from build123d import *

# Parameters (mm, degrees)
SKETCH1_R           = 40
BOSS_EXTRUDE1_DEPTH = 10
CUT_EXTRUDE1_DEPTH  = 4
SKETCH3_W           = 4
SKETCH3_H           = 15
CUT_EXTRUDE2_DEPTH  = 10


with BuildPart() as part:
    # Sketch1 → Boss-Extrude1 (new body)
    with BuildSketch(Plane(origin=(0, 0, 0), x_dir=(1, 0, 0), z_dir=(0, 1, 0))):
        with Locations(Location((0, 0, 0), (0, 0, 270))):
            Circle(SKETCH1_R)
    extrude(amount=BOSS_EXTRUDE1_DEPTH)

    # Sketch2 → Cut-Extrude1 (cut)
    with BuildSketch(Plane(origin=(0, 10, 0), x_dir=(1, 0, 0), z_dir=(0, 1, 0))):
        with BuildLine():
            Line((-2, 16.764144262), (-3.580103784, 0.764144262))
            ThreePointArc((-3.580103784, 0.764144262), (0, -3.596740326), (3.580103784, 0.764144262))
            Line((3.580103784, 0.764144262), (2, 16.764144262))
            ThreePointArc((2, 16.764144262), (0, 18.764144262), (-2, 16.764144262))
        make_face()
    extrude(amount=-CUT_EXTRUDE1_DEPTH, mode=Mode.SUBTRACT)

    # Sketch3 → Cut-Extrude2 (cut)
    with BuildSketch(Plane.XZ):
        with Locations((13, 0)):
            Rectangle(SKETCH3_W, SKETCH3_H)
        with Locations((-13, 0)):
            Rectangle(SKETCH3_W, SKETCH3_H)
    extrude(amount=-CUT_EXTRUDE2_DEPTH, mode=Mode.SUBTRACT)


solid = part.part
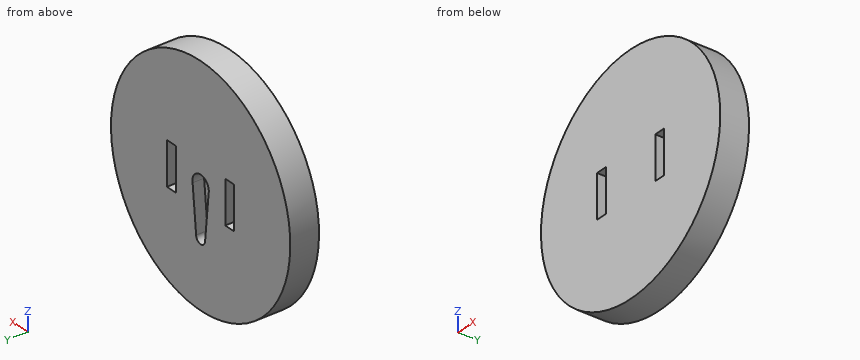
Read the model definition and answer for the solid it produces. Units are mm, in the model's axes. Coordinates: 2 decimals unless noted, no trailing zeros. Write each loop counter-clockwise with the first axis right and the second up, starting at its lowest first coordinate (ties: lowest second). Pieces come first, ordered by that corner, then holes. Notation, with made-up numbers: (29, -36) - (67, -36) arc R21 ccw to (67, -7) - close; hole circle Ø6 at (-3, 4). An arc over 180 degrees is marked (long way). One line per question, with ' | ' between items.
Q1. Find section D-D, the plane z = -5.5. Write down the section's boundary in (x, y), plus the area to 3 significant figures.
Result set:
outline: (-39.62, 0) - (-15, 0) - (-15, 10) - (-39.62, 10) - close; (-11, 0) - (11, 0) - (11, 10) - (3.11, 10) - (3.11, 6) - (-3.11, 6) - (-3.11, 10) - (-11, 10) - close; (15, 0) - (39.62, 0) - (39.62, 10) - (15, 10) - close | area: 688 mm^2
Q2. Find section A-A, the plane y = 3.75. Write down the section's boundary in (x, z).
Result set:
outline: circle Ø80 at (0, 0); hole (-15, -7.5) - (-11, -7.5) - (-11, 7.5) - (-15, 7.5) - close; hole (11, -7.5) - (15, -7.5) - (15, 7.5) - (11, 7.5) - close
Q3. Consider L1, parallel to X at y = 4.5, z = -0.5; L2, parallel to X at y = 1.5, z = 4; L3, parallel to X at y = 8.75, z = 3. Determine where each line is inside the solid, lowest interval first. Write a range as [from, to].
Result set:
L1: [-40, -15], [-11, 11], [15, 40] | L2: [-39.8, -15], [-11, 11], [15, 39.8] | L3: [-39.89, -15], [-11, -2], [2, 11], [15, 39.89]
Q4. Find section C-C, the plane x = 0. Write down the section's boundary in (y, z).
Result set:
outline: (0, -40) - (10, -40) - (10, -18.76) - (6, -18.76) - (6, 3.6) - (10, 3.6) - (10, 40) - (0, 40) - close
Q5. Find section B-B, the plane z = 5. Write down the section's boundary in (x, y), plus the area to 3 significant figures.
Result set:
outline: (-39.69, 0) - (-15, 0) - (-15, 10) - (-39.69, 10) - close; (-11, 0) - (11, 0) - (11, 10) - (-11, 10) - close; (15, 0) - (39.69, 0) - (39.69, 10) - (15, 10) - close | area: 714 mm^2
Q6. Each of these flat-tipped pins is pushed along its axis until it touches: P1, Ø1.5, axis at x = -19, z = -7, coming from the -Y side; P2, Ø4.5, axis at x = -12.5, y = 3, coming from the -Z side; P3, Ø5, axis at y = 4.5, z = 20, coming from the +X side; P4, Ø2, axis at x = -13, y = 5.5, coming from the +Z side. Where does it stop, or does it pass through?
Result set:
P1: y = 0 | P2: z = -38.66 | P3: x = 35.97 | P4: z = 38.16
